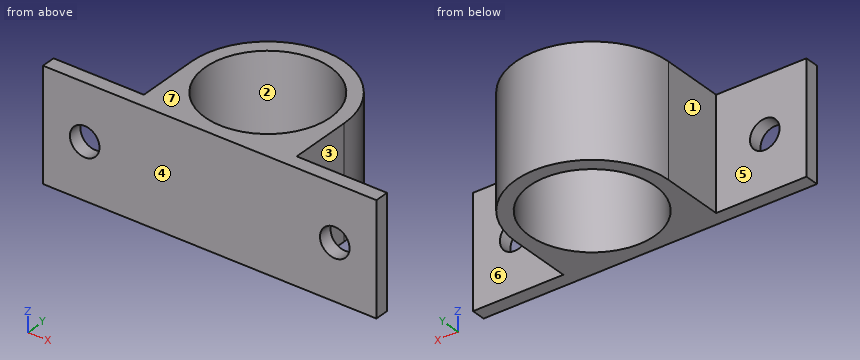
Autodesk Inventor part; units mm, degrees
ref_plane "YZ Plane" through (0, 0, 0) normal (1, 0, 0) x (0, 1, 0)
ref_plane "XZ Plane" through (0, 0, 0) normal (0, 1, 0) x (-1, 0, 0)
ref_plane "XY Plane" through (0, 0, 0) normal (0, 0, 1) x (1, 0, 0)
sketch "Sketch1" plane through (0, 0, 0) normal (0, 0, 1) x (1, 0, 0)
  line L0 (0, 0) -> (-38.1, 0)
  line L1 (0, 0) -> (38.1, 0)
  line L2 (38.1, 0) -> (38.1, 3.175)
  line L3 (38.1, 3.175) -> (-38.1, 3.175)
  line L4 (-38.1, 3.175) -> (-38.1, 0)
  line L5 (0, 0) -> (0, 17.4625)
  circle A0 centre (0, 17.4625) radius 14.2875
  arc A1 (0, 0) -> (0, 0) centre (0, 17.4625) ccw
  circle A2 centre (0, 17.4625) radius 17.4625
  line L6 (-17.4625, 17.4625) -> (-17.4625, 3.175)
  line L7 (17.4625, 17.4625) -> (17.4625, 3.175)
  dimension "d0" = 38.1
  dimension "d1" = 38.1
  dimension "d2" = 3.175
  dimension "d3" = 17.4625
  dimension "d4" = 28.575
  dimension "d16" = 3.175
extrude "Extrusion1" add sketch "Sketch1" along normal blind 25.4 contours A1 L3 L2 L1 | A1 L3 L5 | L0 L4 L3 A1 | L5 L3 A1 | L3 A1
sketch "Sketch2" plane through (19.05, 3.175, 0) normal (0, 1, 0) x (1, 0, 0)
  line L0 (19.05, 0) -> (19.05, -25.4)
  line L1 (19.05, -12.7) -> (9.525, -12.7)
  circle A0 centre (9.525, -12.7) radius 3.3782
  line L2 (-57.15, 0) -> (-57.15, -25.4)
  line L3 (-38.1, 0) -> (-38.1, -25.4)
  line L4 (-57.15, -12.7) -> (-47.625, -12.7)
  circle A1 centre (-47.625, -12.7) radius 3.3782
  point P0 (-19.05, 0)
  dimension "d8" = 6.7564
  dimension "d13" = 9.525
  dimension "d14" = 6.7564
  dimension "d15" = 9.525
extrude "Extrusion2" cut sketch "Sketch2" against normal blind 25.4
sketch "Sketch3" plane through (0, 0, 25.4) normal (0, 0, 1) x (1, 0, 0)
  line L0 (38.1, 3.175) -> (10.0402, 3.175)
  arc A0 (10.0402, 3.175) -> (-10.0402, 3.175) centre (0, 17.4625) ccw
  line L1 (-10.0402, 3.175) -> (-38.1, 3.175)
  line L2 (-17.4625, 17.4625) -> (-17.4625, 3.175)
  line L3 (17.4625, 17.4625) -> (17.4625, 3.175)
  point P0 (0, 0)
extrude "Extrusion3" add sketch "Sketch3" against normal blind 25.4
properties part number "p80 bearing mount" material "Aluminum 6061"
CAD build for the part. Positions are in the model's coordinates, mm. Face numbers are marked on the shaded views. A direction names the side the tool comes from. Coordinates: 2 decimals unless noted, no trailing zeros. Loops run counter-clockwise (first coordinate to the right, second up) from the corner with the lowest first, then second, coordinate; pieces in that order, holes last. Notation, with made-up numbers: (21.5, 34) - (79.5, 34) arc R11 cw to (79.5, 50) - close; hole circle Ø9 at (73, 89). An arc over 180 degrees is marked (long way). Write item = value, one per line. Start each with the question number.
Q1. Cut at A-A, the plane z = 12.7. List the corners of the cut face in (x, y) (1 decimal), then the cut area to 3 significant figures.
Q2. Which spindle directions (+Z, -Z, +X, -X, +Y, -Y) get a long thin tool onto all of the face, cutting with end or side? Do the marked faces 5, 6 and 7. Say none if no direction does.
Q3. Drill centre lines: L1, parallel to X at y = 2.5, z = 12.7; L2, parallel to Y at x = 0, z = 9.75 (3 decimals); L3, parallel to Y at x = 33.5, z = 6.75 (3 decimals). Where is each one in solid material? Low to high.
Q4. Flat gauge pins, fed straight in: pin 1 Ø8 at (y, z) = (9.5, 16.5) entering from +X; pin 2 Ø11 at (x, z) = (28.575, 12.7) entering from +Y (3 decimals); pin 3 Ø3 at (x, y) = (10.5, 31.5) entering from -Z; pin 4 Ø10 at (y, z) = (10.5, 6) entering from -X. Where does each tip first touch, or does it go through?
Q5. Pull direction X, two halves, no side cores. Call the marked faces 1, 2, 3 and 4: pulls with the +X half, pulls with the -X half, needs draft (parallel to the pull), parting line crosses it, or undercut.
Q6. Cut at D-D, the plane y = 14. List the corners of the cut face in (x, z).
Q7. Cut at B-B, the plane x = 0. List the corners of the cut face in (y, z) (3 decimals), then the cut area to 3 significant figures.
Q8. Cut at C-C, the plane z = 7.75. List the corners of the cut face in (x, y) (1 decimal).
Computed:
q1.outline = (-38.1, 0) - (-32, 0) - (-32, 3.2) - (-38.1, 3.2) - close; (-25.2, 0) - (25.2, 0) - (25.2, 3.2) - (17.5, 3.2) - (17.5, 17.5) arc R17.5 ccw to (-17.5, 17.5) - (-17.5, 3.2) - (-25.2, 3.2) - close; (32, 0) - (38.1, 0) - (38.1, 3.2) - (32, 3.2) - close; hole circle Ø28.6 at (0, 17.5)
q1.area = 536 mm²
q2.face_5 = +Z, -Z, -X, +Y
q2.face_6 = +Z, -Z, +X, +Y
q2.face_7 = +Z, +X, -X, +Y, -Y
q3.L1 = -38.1 to -31.95, -25.2 to 25.2, 31.95 to 38.1
q3.L2 = 0 to 3.175, 31.75 to 34.925
q3.L3 = 0 to 3.175
q4.pin_1 = 17.46
q4.pin_2 = 3.175
q4.pin_3 = 0
q4.pin_4 = -17.46
q5.face_1 = pulls with the -X half
q5.face_2 = undercut
q5.face_3 = pulls with the +X half
q5.face_4 = needs draft
q6.outline = (-17.46, 0) - (-13.86, 0) - (-13.86, 25.4) - (-17.46, 25.4) - close; (13.86, 0) - (17.46, 0) - (17.46, 25.4) - (13.86, 25.4) - close
q7.outline = (0, 0) - (3.175, 0) - (3.175, 25.4) - (0, 25.4) - close; (31.75, 0) - (34.925, 0) - (34.925, 25.4) - (31.75, 25.4) - close
q7.area = 161 mm²
q8.outline = (-38.1, 0) - (38.1, 0) - (38.1, 3.2) - (17.5, 3.2) - (17.5, 17.5) arc R17.5 ccw to (-17.5, 17.5) - (-17.5, 3.2) - (-38.1, 3.2) - close; hole circle Ø28.6 at (0, 17.5)
